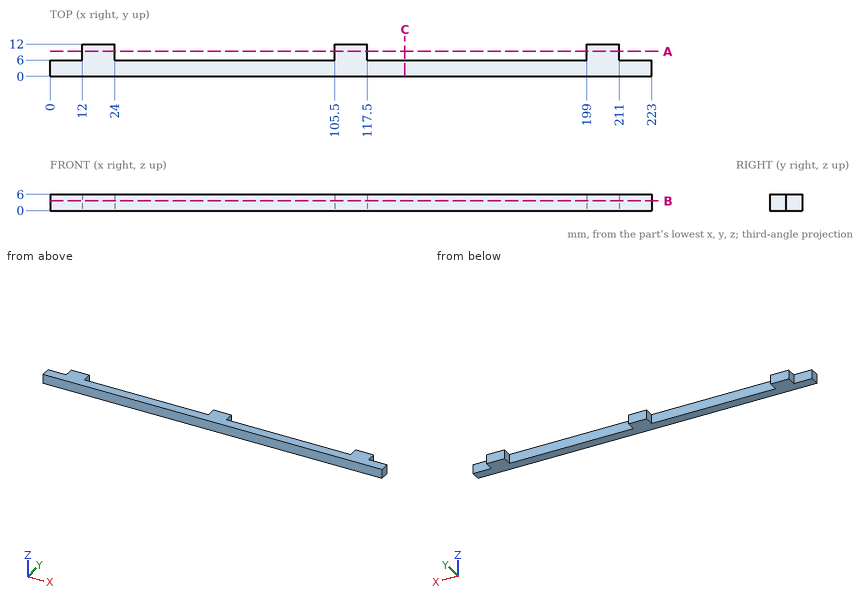
Can you work these out from the drawing? Everything is in mm from the part's minimum corner. Give positions to 0.01 mm unless a question says otherwise; leave off trailing zeros. Order: outer loops, then holes, each group sorted by start corner. A loop starts at its lowest first (then second) coordinate and runs counter-clockwise, first axis right, second up. Notation, with made-up numbers: M 19.25,8.25 L 59.25,8.25 A28 ccw 59.25,40.25 Z; hole C 8.5,85.5 d7. An arc over 180 degrees is marked long. Use a Markdown table: item, result. Add a question column.
1. For pin 1 Ø3 at (x, z) = (215, 1.5) entering from +Y; pin 2 Ø2 at (y, z) = (8.5, 2) entering from -X; pin 3 Ø1.8 at (y, z) = (9.5, 3.5) entering from +X, each with a flat end and sliding along its axis, tell me the tip position at first contact or that it passes through.
2. Suppose I cut it at C-C (x = 131.5). List the corners of the cut face in (y, z) for me, and give its area (3 significant figures).
3. Suppose I cut it at A-A (y = 9.25). List the corners of the cut face in (x, z) for me.
4. I need wall thicknesses on probe 1 along X at (y, z) = (6.25, 5.5); probe 2 along Y at (x, z) = (78, 3.6). Which ranges of each line are inside material? Lowest first, please. Write a range as from..to.
5. Suppose I cut it at B-B (z = 3.6). List the corners of the cut face in (x, y) for me.
Results list:
| question | item | result |
|---|---|---|
| 1 | pin 1 | stops at y = 6 |
| 1 | pin 2 | stops at x = 12 |
| 1 | pin 3 | stops at x = 211 |
| 2 | outline | M 0,0 L 6,0 L 6,6 L 0,6 Z |
| 2 | area | 36.0 mm² |
| 3 | outline | M 12,0 L 24,0 L 24,6 L 12,6 Z; M 105.5,0 L 117.5,0 L 117.5,6 L 105.5,6 Z; M 199,0 L 211,0 L 211,6 L 199,6 Z |
| 4 | probe 1 | x = 12..24, 105.5..117.5, 199..211 |
| 4 | probe 2 | y = 0..6 |
| 5 | outline | M 0,0 L 223,0 L 223,6 L 211,6 L 211,12 L 199,12 L 199,6 L 117.5,6 L 117.5,12 L 105.5,12 L 105.5,6 L 24,6 L 24,12 L 12,12 L 12,6 L 0,6 Z |
